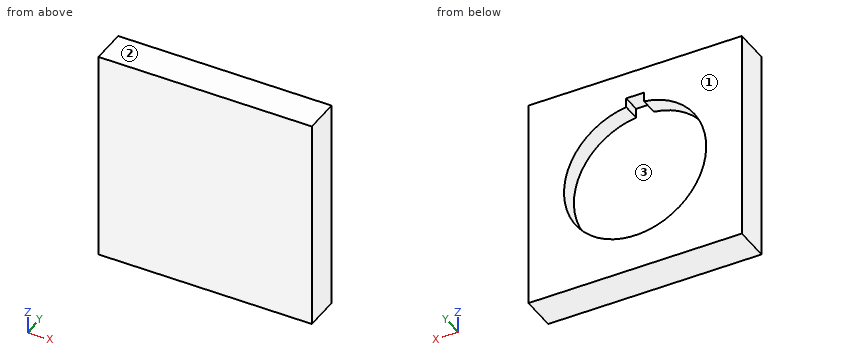
```python
from build123d import *

# Parameters (mm, degrees)
SKETCH1_W           = 152.4
SKETCH1_H           = 152.4
BOSS_EXTRUDE1_DEPTH = 25.4
CUT_EXTRUDE1_DEPTH  = 12.7


with BuildPart() as part:
    # Sketch1 → Boss-Extrude1 (new body)
    with BuildSketch(Plane(origin=(0, 0, 0), x_dir=(1, 0, 0), z_dir=(0, 1, 0))):
        Rectangle(SKETCH1_W, SKETCH1_H)
    extrude(amount=-BOSS_EXTRUDE1_DEPTH)

    # Sketch2 → Cut-Extrude1 (cut)
    with BuildSketch(Plane(origin=(0, 0, 0), x_dir=(1, 0, 0), z_dir=(0, 1, 0))):
        with BuildLine():
            Line((-6.35, -50.401562476), (-6.35, -57.15))
            Line((-6.35, -57.15), (6.35, -57.15))
            Line((6.35, -57.15), (6.35, -50.401562476))
            ThreePointArc((6.35, -50.401562476), (0, 50.8), (-6.35, -50.401562476))
        make_face()
    extrude(amount=-CUT_EXTRUDE1_DEPTH, mode=Mode.SUBTRACT)


solid = part.part
```
Here's how the part is built. I have some questions about the finished solid (model axes, mm). Face numbers are marked on the shaded views. Coordinates: 2 decimals unless noted, no trailing zeros. Order: outer loops, then holes, each group sorted by start corner. A loop starts at its lowest first (then second) coordinate and runs counter-clockwise, first axis right, second up.
Item 1: If we section it at A-A, the plane y = -3: List the corners of the cut face in (x, z) for me, then the cut area to 3 significant figures.
Response values:
outline: (-76.2, -76.2) - (76.2, -76.2) - (76.2, 76.2) - (-76.2, 76.2) - close; hole (-6.35, 50.4) arc R50.8 ccw (long way) to (6.35, 50.4) - (6.35, 57.15) - (-6.35, 57.15) - close
area: 15,000 mm2
Item 2: If we section it at C-C, the plane x = 0: List the corners of the cut face in (y, z) for me.
Response values:
outline: (-25.4, -76.2) - (0, -76.2) - (0, -50.8) - (-12.7, -50.8) - (-12.7, 57.15) - (0, 57.15) - (0, 76.2) - (-25.4, 76.2) - close
Item 3: If we section it at B-B, the plane z = 0: List the corners of the cut face in (x, y) for me, then the cut area to 3 significant figures.
Response values:
outline: (-76.2, -25.4) - (76.2, -25.4) - (76.2, 0) - (50.8, 0) - (50.8, -12.7) - (-50.8, -12.7) - (-50.8, 0) - (-76.2, 0) - close
area: 2,580 mm2
Item 4: I need wall thicknesses on probe 1 along Z at (x, y) = (0, -6.75); probe 2 along X at (y, z) = (-6.5, 0); probe 3 along Y at (x, z) = (23.5, -28.5). Which ranges of each line are inside material? Lowest first, please.
Response values:
probe 1: z = -76.2 to -50.8, 57.15 to 76.2
probe 2: x = -76.2 to -50.8, 50.8 to 76.2
probe 3: y = -25.4 to -12.7
Item 5: Thinking about a two-plate mould opening in Z: for the marked faces 1, 2 and 3, which applies, pulls with the +Z half, pulls with the -Z half, needs draft (parallel to the pull), parting line crosses it, or undercut?
Response values:
face 1: needs draft
face 2: pulls with the +Z half
face 3: undercut
